The listing builds one solid part. Answer for the finished solid, in the listing's coordinates (mm). A direction names the side the tool comes from. Coordinates: 2 decimals unless noted, no trailing zeros. Loops run counter-clockwise (first coordinate to the right, second up) from the corner with the lowest first, then second, coordinate; pieces in that order, holes last. Notation, with made-up numbers: (-8, 40.5) - (-4, 40.5) arc R10 cw to (-4, 52.5) - close; hole circle Ø9 at (58, -4.5). An arc over 180 degrees is marked (long way). Use one line per item in the form item = value. Start each with the question number.
Autodesk Inventor part; units mm, degrees
ref_plane "YZ Plane" through (0, 0, 0) normal (1, 0, 0) x (0, 1, 0)
ref_plane "XZ Plane" through (0, 0, 0) normal (0, 1, 0) x (-1, 0, 0)
ref_plane "XY Plane" through (0, 0, 0) normal (0, 0, 1) x (1, 0, 0)
sketch "Sketch1" plane through (0, 0, 0) normal (0, 1, 0) x (-1, 0, 0)
  line L0 (0, 0) -> (20, 0)
  line L1 (20, 0) -> (20, -50.8)
  line L2 (20, -50.8) -> (70.8, -50.8)
  line L3 (70.8, -50.8) -> (70.8, 0)
  line L4 (70.8, 0) -> (20, 0)
  line L5 (0, 0) -> (0, -70.808)
  line L6 (0, -70.808) -> (90.808, -70.808)
  line L7 (90.808, -70.808) -> (90.808, 20.008)
  line L8 (90.808, 20.008) -> (20, 20.008)
  line L9 (20, 20.008) -> (20, 0)
  dimension "d0" = 20
  dimension "d1" = 50.8
  dimension "d2" = 50.8
  dimension "d3" = 50.8
  dimension "d4" = 50.8
  dimension "d6" = 28.2899
  dimension "d7" = 28.2956
  dimension "d8" = 28.2956
  dimension "d11" = 20.008
extrude "Extrusion1" add sketch "Sketch1" along normal blind 155.0924
properties part number "LegHolder" material "Wood (Birch)"
(1) Determine the mould class of faces 4 (the face through (-20, 76, 10)), 5 (the face through (-46, 76, 0)), 6 (the face through (-75, 0, -25)) for opening direction X: +X half, -X half, draft (parallel to the pull), parting line (faces both ways), or undercut.
(2) A cutting plane is placed at A-A (x = -47). Determine the outline of the cut face in (y, z), then the cut area to 3 significant figures.
(3) A cutting plane is placed at B-B (z = -43). Determine the outline of the cut face in (x, y), then the cut area to 3 significant figures.
(4) A cutting plane is placed at D-D (x = -14.5). Determine the outline of the cut face in (y, z), then the cut area to 3 significant figures.
(5) Each of these flat-tipped pins is pushed along its axis until it touches: pin 1 Ø22 at (y, z) = (45.5, 15) entering from +X; pin 2 Ø10 at (x, y) = (-6.5, 93) entering from +Z; pin 3 Ø15 at (y, z) = (88, -28.5) entering from +X. Where does it stop, or does it pass through?
(6) For faces 1 (the face through (-90.808, 76, -26)), 2 (the face through (-10, 76, 0)), 3 (the face through (-20, 76, -25)), determine the directions among +Z, -Z, +X, -X, +Y, -Y from which every point of the face is accessible in a straight line to the end or side of a thin tool.
(7) Find the intervals of material crossed by probe 1 along Z at (x, y) = (-42.5, 50.5); probe 2 along X at (y, z) = (93.5, -12); probe 3 along Z at (x, y) = (-6, 141), in increasing order. Write a range as from..to.
Evaluation:
q1.face_4 = +X half
q1.face_5 = undercut
q1.face_6 = draft
q2.outline = (0, -70.81) - (155.09, -70.81) - (155.09, -50.8) - (0, -50.8) - close; (0, 0) - (155.09, 0) - (155.09, 20.01) - (0, 20.01) - close
q2.area = 6,210 mm^2
q3.outline = (-90.81, 0) - (-70.8, 0) - (-70.8, 155.09) - (-90.81, 155.09) - close; (-20, 0) - (0, 0) - (0, 155.09) - (-20, 155.09) - close
q3.area = 6,200 mm^2
q4.outline = (0, -70.81) - (155.09, -70.81) - (155.09, 0) - (0, 0) - close
q4.area = 11,000 mm^2
q5.pin_1 = -20
q5.pin_2 = 0
q5.pin_3 = 0
q6.face_1 = +Z, -Z, -X, +Y, -Y
q6.face_2 = +Z, +X, +Y, -Y
q6.face_3 = +Y, -Y
q7.probe_1 = -70.81..-50.8, 0..20.01
q7.probe_2 = -90.81..-70.8, -20..0
q7.probe_3 = -70.81..0
